Check sheet for the modelled part. Datum: model origin and axes. Units: mm. A direction names the side the tool comes from. Coordinates: 2 decimals unless noted, no trailing zeros. Loops run counter-clockwise (first coordinate to the right, second up) from the corner with the lowest first, then second, coordinate; pieces in that order, holes last. Notation, with made-up numbers: (-11, -9.75) -> (-1, -9.75) arc R12 cw to (-1, 8.25) -> close; hole circle Ø4 at (29, -10). An arc over 180 degrees is marked (long way). Use one line per item in the form item = value.
from build123d import *

# Parameters (mm, degrees)
F0_R     = 1.6143877839
F0_R_2   = 1.6384664926
F1_DEPTH = 3


# Not quite as in the source:
# - a feature names something its author has since deleted; it is built from what else it names


with BuildPart() as f1:
    # F0 (on Front) → F1 (new body)
    with BuildSketch(Plane.XZ):
        with BuildLine():
            Line((-39.6336754784, 28), (-39.6336754784, 5))
            ThreePointArc((-39.6336754784, 5), (-38.1692093843, 1.4644660941), (-34.6336754784, 0))
            Line((-34.6336754784, 0), (-18.6336754784, 0))
            ThreePointArc((-18.6336754784, 0), (-15.0981415725, 1.4644660941), (-13.6336754784, 5))
            Line((-13.6336754784, 5), (-13.6336754784, 28))
            ThreePointArc((-13.6336754784, 28), (-15.0981415725, 31.5355339059), (-18.6336754784, 33))
            Line((-18.6336754784, 33), (-34.6336754784, 33))
            ThreePointArc((-34.6336754784, 33), (-38.1692093843, 31.5355339059), (-39.6336754784, 28))
        make_face()
        with Locations((-37.207160145, 16.4869632572)):
            Circle(F0_R, mode=Mode.SUBTRACT)
        Polygon((-34.6336754784, 5), (-34.6336754784, 16.5), (-34.6336754784, 28), (-29.7759659588, 28), (-29.7759659588, 30), (-23.4435740858, 30), (-23.4435740858, 28), (-18.6336754784, 28), (-18.6336754784, 5), align=None, mode=Mode.SUBTRACT)
        with Locations((-16.2413809448, 16.5)):
            Circle(F0_R_2, mode=Mode.SUBTRACT)
    extrude(amount=F1_DEPTH)


solid = f1.part
(1) Go/stop test with a flat-tipped pin: P1, Ø0.6, axis at y = -1, z = 29, coming from the -X side. Record where the tip stops, or that it passes through.
Established:
P1 = -39.58
(2) Section check B-B, the plane x = -19.25. Record the boundary of the cut face in (y, z), plus the area to 3 significant figures.
Established:
outline = (-3, 0) -> (0, 0) -> (0, 5) -> (-3, 5) -> close; (-3, 28) -> (0, 28) -> (0, 33) -> (-3, 33) -> close
area = 30.0 mm²
(3) Tool access check on faces 1 (the flat face through (-21, -1, 28)), 2 (the flat face through (-27, -1, 33)). Record the directions out of +Z, -Z, +X, -X, +Y, -Y that give a thin tool (end or side, any length) a straight path to the whole face; none if there is none.
Established:
face_1 = +Y, -Y
face_2 = +Z, +X, -X, +Y, -Y
(4) Scan lines: line 1 along Z through (x, y) = (-34, -2.9); line 2 along Z through (x, y) = (-25, -1.65); line 3 along X through (y, z) = (-2, 22). Record each from-to range of solid material in increasing order.
Established:
line_1 = 0 to 5, 28 to 33
line_2 = 0 to 5, 30 to 33
line_3 = -39.63 to -34.63, -18.63 to -13.63
(5) Mould release check, pull along X, two halves, no side actions. Record for faces 3 (the flat face through (-29.776, -1, 29)), 4 (the flat face through (-27, -1, 0)), 5 (the flat face through (-23.444, -1, 29)), 6 (the cylindrical face through (-38.13, -1.479, 31.574)): +X half, -X half, draft (parallel to the pull), parting line (faces both ways), or undercut.
Established:
face_3 = undercut
face_4 = draft
face_5 = undercut
face_6 = -X half
(6) Section check A-A, the plane z = 25.5. Record the boundary of the cut face in (x, y).
Established:
outline = (-39.63, -3) -> (-34.63, -3) -> (-34.63, 0) -> (-39.63, 0) -> close; (-18.63, -3) -> (-13.63, -3) -> (-13.63, 0) -> (-18.63, 0) -> close
(7) Section check C-C, the plane y = -0.6. Record the boundary of the cut face in (x, z).
Established:
outline = (-39.63, 5) arc R5 ccw to (-34.63, 0) -> (-18.63, 0) arc R5 ccw to (-13.63, 5) -> (-13.63, 28) arc R5 ccw to (-18.63, 33) -> (-34.63, 33) arc R5 ccw to (-39.63, 28) -> close; hole circle Ø3.23 at (-37.21, 16.49); hole (-34.63, 5) -> (-18.63, 5) -> (-18.63, 28) -> (-23.44, 28) -> (-23.44, 30) -> (-29.78, 30) -> (-29.78, 28) -> (-34.63, 28) -> close; hole circle Ø3.28 at (-16.24, 16.5)
